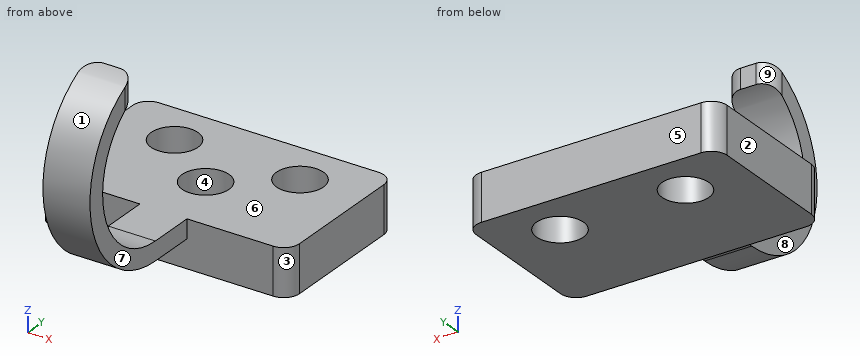
from build123d import *

# Parameters (mm, degrees)
F0_W      = 101.6
F0_H      = 63.5
F1_DEPTH  = 19.05
F2_R      = 6.35
F3_R      = 9.525
F4_DEPTH  = 12.7
F5_DEPTH  = 19.051
F6_W      = 19.05
F6_H      = 7.62
F7_DEPTH  = 19.05
F8_W      = 19.05
F8_H      = 7.62
F9_ANGLE  = 162.2017998475
F11_DEPTH = 25.4
F12_R     = 6.35


with BuildPart() as f1:
    # F0 (on Top) → F1 (new body)
    with BuildSketch(Plane.XY):
        with Locations((50.8, -31.75)):
            Rectangle(F0_W, F0_H)
    extrude(amount=F1_DEPTH)

    # F2
    f2_edges = [f1.edges().sort_by_distance(p)[0] for p in [
        (101.6, -63.5, 9.525),
        (101.6, 0, 9.525),
        (0, -63.5, 9.525),
        (0, 0, 9.525),
    ]]
    fillet(f2_edges, radius=F2_R)

    # F3 (on face) → F4 (cut)
    with BuildSketch(Plane.XY.offset(19.05)):
        with Locations((50.8, -38.1)):
            Circle(F3_R)
    extrude(amount=-F4_DEPTH, mode=Mode.SUBTRACT)

    # F3 (on face) → F5 (cut, through all)
    with BuildSketch(Plane.XY.offset(19.05)):
        with Locations((25.4, -19.05)):
            Circle(F3_R)
        with Locations((76.2, -19.05)):
            Circle(F3_R)
    extrude(amount=-F5_DEPTH, mode=Mode.SUBTRACT)

    # F6 (on face) → F7 (join)
    with BuildSketch(Plane.XZ.offset(63.5)):
        with Locations((50.8, 15.24)):
            Rectangle(F6_W, F6_H)
    extrude(amount=F7_DEPTH)

    # F8 (on face) → F9 (revolve)
    with BuildSketch(Plane.XZ.offset(82.55)):
        with Locations((50.8, 15.24)):
            Rectangle(F8_W, F8_H)
    revolve(axis=Axis((50.8, -82.55, 50.8), (-1, 0, 0)), revolution_arc=F9_ANGLE)

    # F10 (on face) → F11 (cut)
    with BuildSketch(Plane.YZ.offset(60.325)):
        with BuildLine():
            Line((-94.5840466137, 88.2857122395), (-94.5840466137, 80.1810180576))
            ThreePointArc((-94.5840466137, 80.1810180576), (-93.4277552997, 80.6284585529), (-92.2548763014, 81.0304130963))
            Line((-92.2548763014, 81.0304130963), (-94.5840466137, 88.2857122395))
        make_face()
        with BuildLine():
            Line((-86.6367444396, 76.66990906), (-86.6367444396, 88.2857122395))
            Line((-86.6367444396, 88.2857122395), (-94.5840466137, 88.2857122395))
            Line((-94.5840466137, 88.2857122395), (-92.2548763014, 81.0304130963))
            ThreePointArc((-92.2548763014, 81.0304130963), (-93.4277552997, 80.6284585529), (-94.5840466137, 80.1810180576))
            Line((-94.5840466137, 80.1810180576), (-94.5840466137, 76.66990906))
            Line((-94.5840466137, 76.66990906), (-86.6367444396, 76.66990906))
        make_face()
    extrude(amount=-F11_DEPTH, mode=Mode.SUBTRACT)

    # F12
    f12_edges = [f1.edges().sort_by_distance(p)[0] for p in [
        (60.325, -94.584047, 84.233365),
        (41.275, -94.584047, 84.233365),
    ]]
    fillet(f12_edges, radius=F12_R)


solid = f1.part
Model file for the job. Use its own axes, mm. Face numbers are marked on the shaded views. A direction names the side the tool comes from. Coordinates: 2 decimals unless noted, no trailing zeros. Write each loop counter-clockwise with the first axis right and the second up, starting at its lowest first coordinate (ties: lowest second). Pieces come first, ordered by that corner, then holes. Notation, with made-up numbers: (68.5, -24) - (77.5, -24) arc R25 cw to (77.5, 3) - close; hole circle Ø5 at (70.25, 9.5). An arc over 180 degrees is marked (long way). Write each question's results on one line, items separated by ' | '. Start each with the question number.
1) Probe line 1 along X through (y, z) = (-19, 6); line 2 along Y through (x, z) = (50.8, 11.25) (3 decimals); line 3 along Y through (x, z) = (50.8, 16) (3 decimals). List the from-to ranges inside material, lowest first. Write a range as from..to.
2) Mould opens along X. For the marked faces 1, 2, 3 and 4 say: pulls with the +X half, pulls with the -X half, needs draft (parallel to the pull), parting line crosses it, or undercut.
3) Cut at C-C (y = -38.1). Write the cut outline in (x, z) (3 decimals), then the cut area to 3 significant figures.
4) 3-axis set-ups, long thin cutter, end or side, ignore diameter. For the marked faces 5, 6, 7, 8 and 9: which of +Z, -Z, +X, -X, +Y, -Y reach the whole face in a straight line?
5) Cut at A-A (y = -19.05). Write the cut outline in (x, z) (3 decimals).
6) Cut at D-D (x = 50.8). Write the cut outline in (y, z) (3 decimals), then the cut area to 3 significant figures.
7) Flat gauge pins, fed straight in: P1, Ø3, axis at x = 49.5, z = 83, coming from the +Y side; P2, Ø5, axis at x = 51.5, z = 42, coming from the +Y side; P3, Ø15, axis at x = 42.5, z = 8.5, coming from the -Y side. Where does each tip first touch, or does it go through?
8) Cut at B-B (x = 25.4). Write the cut outline in (y, z) (3 decimals), then the cut area to 3 significant figures.
Returned:
1) line 1: 0..15.88, 34.92..66.68, 85.72..101.6 | line 2: -63.5..-47.625, -28.575..0 | line 3: -100.961..-47.625, -28.575..0
2) face 1: needs draft | face 2: pulls with the -X half | face 3: pulls with the +X half | face 4: undercut
3) outline: (0, 0) - (101.6, 0) - (101.6, 19.05) - (60.325, 19.05) - (60.325, 6.35) - (41.275, 6.35) - (41.275, 19.05) - (0, 19.05) - close | area: 1,690 mm^2
4) face 5: +Z, -Z, +X, -X, +Y | face 6: +Z, +X, -X, +Y | face 7: +Z, -Z, +X, -Y | face 8: +Z, -Z, -X, -Y | face 9: +Z, -X, +Y
5) outline: (0, 0) - (15.875, 0) - (15.875, 19.05) - (0, 19.05) - close; (34.925, 0) - (66.675, 0) - (66.675, 19.05) - (34.925, 19.05) - close; (85.725, 0) - (101.6, 0) - (101.6, 19.05) - (85.725, 19.05) - close
6) outline: (-94.584, 80.181) - (-94.584, 88.286) arc R39.37 ccw to (-82.55, 11.43) - (-63.5, 11.43) - (-63.5, 0) - (0, 0) - (0, 19.05) - (-28.575, 19.05) - (-28.575, 6.35) - (-47.625, 6.35) - (-47.625, 19.05) - (-82.55, 19.05) arc R31.75 cw to start | area: 1,870 mm^2
7) P1: y = -94.58 | P2: y = -112.22 | P3: y = -100.96
8) outline: (-63.5, 0) - (-28.575, 0) - (-28.575, 19.05) - (-63.5, 19.05) - close; (-9.525, 0) - (0, 0) - (0, 19.05) - (-9.525, 19.05) - close | area: 847 mm^2
